Job drawing, mm, ordinate dimensions from the low corner. One solid piece. Give positions to 0.01 mm unless a question says otherwise; leave off trailing zeros. Order: outer loops, then holes, each group sorted by start corner. A loop starts at its lowest first (then second) coordinate and runs counter-clockwise, first axis right, second up.
Item 1: Band-saw the part on A-A on y = 38.1. Give the cut face in (x, z), plus the area to 3 significant figures.
Item 2: Band-saw the part on B-B on x = 165.1. Give the cut face in (y, z).
Item 3: Band-saw the part on D-D on x = 12.7. Give the cut face in (y, z).
Item 4: Band-saw the part on C-C on z = 2. Count the separate pieces of the cut face and the enclosed holes in it, plus the area to 3 significant figures.
Item 5: Flat gauge pin, fed straight in: P1, Ø3, axis at x = 165.1, y = 88.9, coming from the +Z side. Where does the tip first touch, or does it go through?
Item 6: Wall check: L1, parallel to Y at x = 63, z = 1.75; L2, parallel to Y at x = 33, z = 3.25; L3, parallel to X at y = 76, z = 5.5. Give the ranges that are in metal, low to high.
Item 7: Two-plate mould, pull along Z, no slides. Class the marked faces 1 and 2: released by +Z, released by -Z, zero draft, split by the parting line, or undercut.
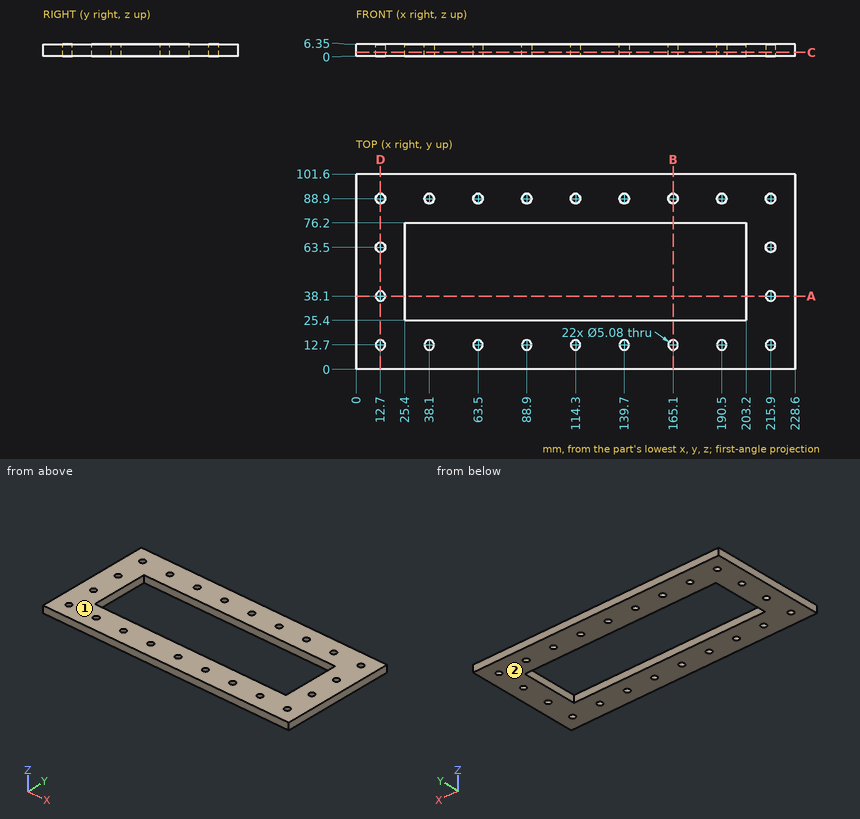
The answers:
1. outline: (0, 0) - (10.16, 0) - (10.16, 6.35) - (0, 6.35) - close; (15.24, 0) - (25.4, 0) - (25.4, 6.35) - (15.24, 6.35) - close; (203.2, 0) - (213.36, 0) - (213.36, 6.35) - (203.2, 6.35) - close; (218.44, 0) - (228.6, 0) - (228.6, 6.35) - (218.44, 6.35) - close
1. area: 258 mm2
2. outline: (0, 0) - (10.16, 0) - (10.16, 6.35) - (0, 6.35) - close; (15.24, 0) - (25.4, 0) - (25.4, 6.35) - (15.24, 6.35) - close; (76.2, 0) - (86.36, 0) - (86.36, 6.35) - (76.2, 6.35) - close; (91.44, 0) - (101.6, 0) - (101.6, 6.35) - (91.44, 6.35) - close
3. outline: (0, 0) - (10.16, 0) - (10.16, 6.35) - (0, 6.35) - close; (15.24, 0) - (35.56, 0) - (35.56, 6.35) - (15.24, 6.35) - close; (40.64, 0) - (60.96, 0) - (60.96, 6.35) - (40.64, 6.35) - close; (66.04, 0) - (86.36, 0) - (86.36, 6.35) - (66.04, 6.35) - close; (91.44, 0) - (101.6, 0) - (101.6, 6.35) - (91.44, 6.35) - close
4. separate pieces: 1
4. enclosed holes: 23
4. area: 13,700 mm2
5. P1: passes through
6. L1: y = 0 to 10.21, 15.19 to 25.4, 76.2 to 86.41, 91.39 to 101.6
6. L2: y = 0 to 25.4, 76.2 to 101.6
6. L3: x = 0 to 25.4, 203.2 to 228.6
7. face 1: released by +Z
7. face 2: released by -Z
